Input: part model. Units: mm. Frame: model coordinates. A direction names the side the tool comes from. Coordinates: 2 decimals unless noted, no trailing zeros. Write each loop counter-clockwise with the first axis right and the second up, starting at its lowest first coordinate (ties: lowest second). Pieces come first, ordered by that corner, then holes. Notation, with made-up numbers: (-38.75, 60.25) - (-21.75, 60.25) arc R9 cw to (-21.75, 69.25) - close; hole circle Ø3 at (26.5, 66.25). An arc over 180 degrees is marked (long way). Put each result on its own line as item: value. Start each with the question number.
1. Pin query (flat end, axial travel): pin 1 (4 mm diameter, centred on x = 27.5, y = 0, fed in from +Z); pin 2 (5 mm diameter, centred on x = 22.5, z = 18, fed in from -Y); pin 3 (12 mm diameter, centred on y = 15.5, z = 22, fed in from -X); pin 4 (0.8 mm diameter, centred on x = 0, y = 25, fed in from -Z). Return the tip coordinate at first contact, or that it passes through.
2. Cut plane D-D, the plane z = 21. Return loops of the section in (x, y), and give its area (3 significant figures).
3. Line query: line 1 (Y direction, x = 0, z = -2); line 2 (Y direction, x = -27.5, z = -1.3); line 3 (Z direction, x = -3.5, y = -31). Output: solid intervals per line, ascending.
4. Cut plane A-A, the plane x = -27.5. Return loops of the section in (y, z), and give its area (3 significant figures).
5. Pull-direction query (X, two-part tool) for faces 1 (the cylindrical face through (-0.417, 30.673, -1.479)), 2 (the flat face through (14, -14, 0)), 3 (the cylindrical face through (-22.3, 11.3, 18.2)); classes: released by +X, released by -X, zero draft, split by the parting line, or undercut.
6. Access query for faces 4 (the flat face through (14.126, -16.919, 18.241)), 5 (the flat face through (22, 0, 18)), 6 (the flat face through (0, 0, 34)), 7 (the flat face through (0, 20, -3)). Directions: +Z, -Z, +X, -X, +Y, -Y. A direction counts if a zero-diameter tool reaches every point of the face in a straight line with its end or side. Return the directions, or none.
7. Cut plane B-B, the plane y = 27.5. Return loops of the section in (x, z), and give its area (3 significant figures).
8. Cut plane C-C, the plane x = -18. Return loops of the section in (y, z).
from build123d import *

# Parameters (mm, degrees)
ESQUISSE1_R                  = 25
BOSS_EXTRU_1_DEPTH           = 37
ENL_V_MAT_EXTRU_1_DEPTH      = 3
ENL_V_MAT_EXTRU_1_DEPTH_BACK = 34
ESQUISSE4_R                  = 19
ENL_V_MAT_EXTRU_3_DEPTH      = 52.176166328
ESQUISSE9_R                  = 37.5
BOSS_EXTRU_2_DEPTH           = 3
ENL_V_START                  = 3
ESQUISSE4_2_R                = 19
ENL_V_MAT_EXTRU_4_DEPTH      = 3
D_GAGEMENT_M61_D             = 6.4
D_GAGEMENT_M61_DEPTH         = 3
ENL_V_START_2                = -3
ENL_V_MAT_EXTRU_5_DEPTH      = 3
CONG_1_R                     = 10
CONG_1_OF_SYM_TRIE4_R        = 10
SYM_TRIE5_START              = -3
SYM_TRIE5_DEPTH              = 3


# Read off the part's stored shape, not the designer's step: Symétrie5
with BuildPart() as part:
    # Esquisse1 → Boss.-Extru.1 (new body)
    with BuildSketch(Plane.XY):
        Circle(ESQUISSE1_R)
    extrude(amount=BOSS_EXTRU_1_DEPTH)

    # Esquisse4 → Enlèv. mat.-Extru.1 (cut, two sides: drawn at the far end of the back side and taken through both)
    with BuildSketch(Plane(origin=(0, 0, 0), x_dir=(-1, 0, 0), z_dir=(0, 0, -1)).offset(-ENL_V_MAT_EXTRU_1_DEPTH_BACK)):
        with Locations(Location((0, 0, 0), (0, 0, 180))):
            Circle(ESQUISSE4_R)
    extrude(amount=ENL_V_MAT_EXTRU_1_DEPTH + ENL_V_MAT_EXTRU_1_DEPTH_BACK, mode=Mode.SUBTRACT)

    # Esquisse7 → Enlèv. mat.-Extru.3 (cut, through all)
    with BuildSketch(Plane(origin=(0, 0, 0), x_dir=(-1, 0, 0), z_dir=(0, 0, -1))):
        with BuildLine():
            Line((-16.192810305, -19.047122996), (-11.999578126, -14.731263517))
            ThreePointArc((-11.999578126, -14.731263517), (-17.160885531, -8.154998946), (-19, 0))
            Line((-19, 0), (-25, 0))
            ThreePointArc((-25, 0), (-22.69163125, -10.492372048), (-16.192810305, -19.047122996))
        make_face()
    extrude(amount=-ENL_V_MAT_EXTRU_3_DEPTH, mode=Mode.SUBTRACT)

    # Esquisse9 → Boss.-Extru.2 (add)
    with BuildSketch(Plane(origin=(0, 0, 0), x_dir=(-1, 0, 0), z_dir=(0, 0, -1))):
        Circle(ESQUISSE9_R)
    extrude(amount=BOSS_EXTRU_2_DEPTH)

    # Esquisse4<2> → Enlèv. mat.-Extru.4 (cut)
    with BuildSketch(Plane(origin=(0, 0, 0), x_dir=(-1, 0, 0), z_dir=(0, 0, -1)).offset(ENL_V_START)):
        with Locations(Location((0, 0, 0), (0, 0, 180))):
            Circle(ESQUISSE4_2_R)
    extrude(amount=-ENL_V_MAT_EXTRU_4_DEPTH, mode=Mode.SUBTRACT)

    # Dégagement M61
    with Locations(Plane(origin=(0, 0, -3), x_dir=(-1, 0, 0), z_dir=(0, 0, -1))):
        with Locations((0, 27.5), (27.5, 0), (0, -27.5), (-27.5, 0)):
            Hole(D_GAGEMENT_M61_D / 2, depth=D_GAGEMENT_M61_DEPTH)

    # Esquisse15 → Enlèv. mat.-Extru.5 (cut)
    with BuildSketch(Plane(origin=(0, 0, -3), x_dir=(-1, 0, 0), z_dir=(0, 0, -1)).offset(ENL_V_START_2)):
        with BuildLine():
            Line((34.932786702, 13.636363636), (25.617376915, 10))
            ThreePointArc((25.617376915, 10), (19.384796538, 19.505887911), (9.840281362, 25.679152297))
            Line((9.840281362, 25.679152297), (12.051640076, 35.51067405))
            ThreePointArc((12.051640076, 35.51067405), (25.913422274, 27.106171734), (34.932786702, 13.636363636))
        make_face()
    enl_v_mat_extru_5 = extrude(amount=ENL_V_MAT_EXTRU_5_DEPTH, mode=Mode.SUBTRACT)

    # Congé1
    # the kernel refuses this fillet: 10 mm, written as the material it takes off along each edge
    with BuildSketch(Plane(origin=(-12.051640076, 35.51067405, 30.511737931), x_dir=(0.9866266204606564, 0.16299666192405335, 0), z_dir=(0, 0, -1))) as cong_1_piece_1:
        with BuildLine():
            CenterArc((10.577402483, 9.866707582), CONG_1_R, 178.889666711, 100.475681696)
            Line((0.579280147, 10.060485169), (0.3793177, 10.064360721))
            ThreePointArc((0.3793177, 10.064360721), (0.089970794, 5.04173949), (-0.199669279, 0.011496906))
            Line((-0.199669279, 0.011496906), (-0.032545854, -0.197334152))
            ThreePointArc((-0.032545854, -0.197334152), (6.102347586, -0.699846569), (12.237241026, -0.197334152))
            Line((12.237241026, -0.197334152), (12.204695172, 0))
        make_face()
    extrude(amount=64.023475862, mode=Mode.SUBTRACT)
    with BuildSketch(Plane(origin=(-34.932786702, 13.636363636, 34.090909091), x_dir=(-0.18820424606330075, -0.9821299108385533, 0), z_dir=(0, 0, -1))) as cong_1_piece_2:
        with BuildLine():
            CenterArc((11.818181818, -9.83332166), CONG_1_R, 79.524318304, 100.475681696)
            Line((1.818181818, -9.83332166), (1.618181818, -9.83332166))
            ThreePointArc((1.618181818, -9.83332166), (0.712424476, -4.953024467), (-0.196666433, -0.036363636))
            Line((-0.196666433, -0.036363636), (-0.036363636, 0.196666433))
            ThreePointArc((-0.036363636, 0.196666433), (6.818181818, 0.825043774), (13.672727273, 0.196666433))
            Line((13.672727273, 0.196666433), (13.636363636, 0))
        make_face()
    extrude(amount=71.181818182, mode=Mode.SUBTRACT)

    # Symétrie4: Enlèv. mat.-Extru.5 across plane
    add(enl_v_mat_extru_5.mirror(Plane(origin=(0, 0, 0), x_dir=(0, 0, 1), z_dir=(1, 0, 0))), mode=Mode.SUBTRACT)

    # Congé1 of Symétrie4
    # the kernel refuses this fillet: 10 mm, written as the material it takes off along each edge
    with BuildSketch(Plane(origin=(12.051640076, 35.51067405, 30.511737931), x_dir=(-0.9866266204606562, 0.1629966619240532, 0), z_dir=(0, 0, -1))) as cong_1_of_sym_trie4_piece_1:
        with BuildLine():
            CenterArc((10.577402483, -9.866707582), CONG_1_OF_SYM_TRIE4_R, 80.634651593, 100.475681696)
            Line((0.579280147, -10.060485169), (0.3793177, -10.064360721))
            ThreePointArc((0.3793177, -10.064360721), (0.089970794, -5.04173949), (-0.199669279, -0.011496906))
            Line((-0.199669279, -0.011496906), (-0.032545854, 0.197334152))
            ThreePointArc((-0.032545854, 0.197334152), (6.102347586, 0.699846569), (12.237241026, 0.197334152))
            Line((12.237241026, 0.197334152), (12.204695172, 0))
        make_face()
    extrude(amount=64.023475862, mode=Mode.SUBTRACT)
    with BuildSketch(Plane(origin=(34.932786702, 13.636363636, 34.090909091), x_dir=(0.18820424606330144, -0.982129910838553, 0), z_dir=(0, 0, -1))) as cong_1_of_sym_trie4_piece_2:
        with BuildLine():
            CenterArc((11.818181818, 9.83332166), CONG_1_OF_SYM_TRIE4_R, 180, 100.475681696)
            Line((1.818181818, 9.83332166), (1.618181818, 9.83332166))
            ThreePointArc((1.618181818, 9.83332166), (0.712424476, 4.953024467), (-0.196666433, 0.036363636))
            Line((-0.196666433, 0.036363636), (-0.036363636, -0.196666433))
            ThreePointArc((-0.036363636, -0.196666433), (6.818181818, -0.825043774), (13.672727273, -0.196666433))
            Line((13.672727273, -0.196666433), (13.636363636, 0))
        make_face()
    extrude(amount=71.181818182, mode=Mode.SUBTRACT)

    # Symétrie5 outline → Symétrie5 (cut)
    with BuildSketch(Plane.XY.offset(SYM_TRIE5_START)):
        with BuildLine():
            ThreePointArc((-0.010162924, -37.499998623), (-7.696247071, -33.893936965), (-9.840281362, -25.679152297))
            ThreePointArc((-9.840281362, -25.679152297), (-19.384796538, -19.505887911), (-25.617376915, -10))
            ThreePointArc((-25.617376915, -10), (-33.845353653, -7.907162456), (-37.499208239, -0.243683034))
            ThreePointArc((-37.499208239, -0.243683034), (-26.433813461, -26.59893806), (-0.010162924, -37.499998623))
        make_face()
        with BuildLine():
            ThreePointArc((9.840281362, -25.679152297), (7.696247071, -33.893936965), (0.010162924, -37.499998623))
            ThreePointArc((0.010162924, -37.499998623), (26.433813461, -26.59893806), (37.499208239, -0.243683034))
            ThreePointArc((37.499208239, -0.243683034), (33.845353653, -7.907162456), (25.617376915, -10))
            ThreePointArc((25.617376915, -10), (19.384796538, -19.505887911), (9.840281362, -25.679152297))
        make_face()
    extrude(amount=SYM_TRIE5_DEPTH, mode=Mode.SUBTRACT)


solid = part.part
Report:
1. pin 1: passes through
1. pin 2: stops at y = 0
1. pin 3: stops at x = -23.12
1. pin 4: stops at z = 0
2. outline: (12, -14.73) arc R19 cw (long way) to (19, 0) - (25, 0) arc R25 ccw (long way) to (16.19, -19.05) - close
2. area: 714 mm^2
3. line 1: y = -37.5 to -30.7, -24.3 to -19, 19 to 24.3, 30.7 to 37.5
3. line 2: y = -10.18 to -3.2, 3.2 to 10.18
3. line 3: z = -3 to 0
4. outline: (-10.18, -3) - (-3.2, -3) - (-3.2, 0) - (-10.18, 0) - close; (3.2, -3) - (10.18, -3) - (10.18, 0) - (3.2, 0) - close
4. area: 41.9 mm^2
5. face 1: undercut
5. face 2: zero draft
5. face 3: split by the parting line
6. face 4: +Z, +X
6. face 5: +Z, +X, -Y
6. face 6: -Z
6. face 7: -Z, +X, -X, +Y, -Y
7. outline: (-10.01, -3) - (-3.2, -3) - (-3.2, 0) - (-10.01, 0) - close; (3.2, -3) - (10.01, -3) - (10.01, 0) - (3.2, 0) - close
7. area: 40.8 mm^2
8. outline: (-20.79, -3) - (-6.08, -3) - (-6.08, 34) - (6.08, 34) - (6.08, -3) - (20.79, -3) - (20.79, 0) - (17.35, 0) - (17.35, 37) - (-17.35, 37) - (-17.35, 0) - (-20.79, 0) - close
